```python
from build123d import *

# Parameters (mm, degrees)
DODANIE_WYCI_GNI_CIE1_DEPTH = 7
SZKIC2_OUTSIDE_W            = 61.616
SZKIC2_OUTSIDE_H            = 65.792
SZKIC2_OUTSIDE_R            = 13.5
WYTNIJ_WYCI_GNI_CIE1_DEPTH  = 7
WYTNIJ_WYCI_GNI_CIE1_TAPER  = 60
SZKIC3_R                    = 10.48
DODANIE_WYCI_GNI_CIE2_DEPTH = 25
SZKIC4_R                    = 7.25
WYTNIJ_WYCI_GNI_CIE2_DEPTH  = 20
SZKIC5_R                    = 3.75
WYTNIJ_WYCI_GNI_CIE3_DEPTH  = 12
SFAZOWANIE1_SIZE            = 1.5


with BuildPart() as part:
    # Szkic1 → Dodanie-wyciągnięcie1 (new body)
    with BuildSketch(Plane(origin=(0, 0, 0), x_dir=(0, 0, -1), z_dir=(1, 0, 0))):
        Polygon((13.5, 7.794228634), (0, 15.588457268), (-13.5, 7.794228634), (-13.5, -7.794228634), (0, -15.588457268), (13.5, -7.794228634), align=None)
    extrude(amount=-DODANIE_WYCI_GNI_CIE1_DEPTH)

    # Szkic2 outside → Wytnij-wyciągnięcie1 (cut)
    with BuildSketch(Plane(origin=(0, 0, 0), x_dir=(0, 0, -1), z_dir=(1, 0, 0))):
        Rectangle(SZKIC2_OUTSIDE_W, SZKIC2_OUTSIDE_H)
        Circle(SZKIC2_OUTSIDE_R, mode=Mode.SUBTRACT)
    extrude(amount=-WYTNIJ_WYCI_GNI_CIE1_DEPTH, taper=WYTNIJ_WYCI_GNI_CIE1_TAPER, mode=Mode.SUBTRACT)

    # Szkic3 → Dodanie-wyciągnięcie2 (add)
    with BuildSketch(Plane.ZY.offset(7)):
        Circle(SZKIC3_R)
    extrude(amount=DODANIE_WYCI_GNI_CIE2_DEPTH)

    # Szkic4 → Wytnij-wyciągnięcie2 (cut)
    with BuildSketch(Plane.ZY.offset(32)):
        Circle(SZKIC4_R)
    extrude(amount=-WYTNIJ_WYCI_GNI_CIE2_DEPTH, mode=Mode.SUBTRACT)

    # Szkic5 → Wytnij-wyciągnięcie3 (cut)
    with BuildSketch(Plane(origin=(0, 0, 0), x_dir=(0, 0, -1), z_dir=(1, 0, 0))):
        Circle(SZKIC5_R)
    extrude(amount=-WYTNIJ_WYCI_GNI_CIE3_DEPTH, mode=Mode.SUBTRACT)

    # Sfazowanie1
    sfazowanie1_edges = [part.edges().sort_by_distance(p)[0] for p in [
        (-32, 0, -10.48),
    ]]
    chamfer(sfazowanie1_edges, length=SFAZOWANIE1_SIZE)

    # Szkic6 → Wycięcie-obrót1 (revolve, cut)
    with BuildSketch(Plane.XY):
        with BuildLine():
            Line((-9, 10), (-9, 11.5))
            Line((-9, 11.5), (-7, 11.5))
            Line((-7, 11.5), (-7, 10))
            ThreePointArc((-7, 10), (-8, 9), (-9, 10))
        make_face()
    revolve(axis=Axis((0, 0, 0), (-1, 0, 0)), mode=Mode.SUBTRACT)


solid = part.part
```
The listing builds one solid part. Answer for the finished solid, in the listing's coordinates (mm). A direction names the side the tool comes from. Give positions to 0.01 mm unless a question says otherwise; leave off trailing zeros. Order: outer loops, then holes, each group sorted by start corner. A loop starts at its lowest first (then second) coordinate and runs counter-clockwise, first axis right, second up. Notation, with made-up numbers: (7.5, 2.5) -> (21.5, 2.5) arc R32 cw to (21.5, 34.5) -> close; hole circle Ø1 at (68.25, -34). An arc over 180 degrees is marked (long way). Answer as CSV lines item,"result". Start each with the question number.
Q1. Which of the six approach directions +Z, -Z, +X, -X, +Y, -Y give full straight-line access (tool end or side, diameter ignored) to faces 1 (the conical face through (-0.29, 7.03, -12.11)), 2 (the cylindrical face through (-19.6, 10.39, -1.36))?
Q2. A cutting plane is placed at A-A (x = -3). Determine the outline of the cut face in (y, z), then the cut area to 3 significant figures.
Q3. Given pin 1 (8 mm diameter, centred on y = 2.5, z = -1.5, fed in from -X); pin 2 (2 mm diameter, centred on x = -9, z = -4.5, fed in from -Y); pin 3 (10 mm diameter, centred on x = -23, z = -3.5, fed in from +Y), each flat-ended and moving along its own axis, determine where each tip first touches the part or whether it passes through.
Q4. A cutting plane is placed at B-B (x = -17). Determine the outline of the cut face in (y, z), then the cut area to 3 significant figures.
Q5. Find the intervals of material crossed by L1, parallel to Y at x = -3, z = 0; L2, parallel to Y at x = -24.25, z = 0; L3, parallel to X at y = -5, z = -1, in increasing order.
Results found:
1,face 1,"-Z, +X, +Y"
1,face 2,"-X"
2,outline,"(-15.59, 0) -> (-7.79, -13.5) -> (7.79, -13.5) -> (15.59, 0) -> (7.79, 13.5) -> (-7.79, 13.5) -> close; hole circle Ø7.5 at (0, 0)"
2,area,"587 mm2"
3,pin 1,"x = -12"
3,pin 2,"y = -9.88"
3,pin 3,"y = 10.48"
4,outline,"circle Ø20.96 at (0, 0); hole circle Ø14.5 at (0, 0)"
4,area,"180 mm2"
5,L1,"-15.59 to -3.75, 3.75 to 15.59"
5,L2,"-10.48 to -7.25, 7.25 to 10.48"
5,L3,"-12 to 0"
